Autodesk Inventor part; units mm, degrees
ref_plane "YZ Plane" through (0, 0, 0) normal (1, 0, 0) x (0, 1, 0)
ref_plane "XZ Plane" through (0, 0, 0) normal (0, 1, 0) x (-1, 0, 0)
ref_plane "XY Plane" through (0, 0, 0) normal (0, 0, 1) x (1, 0, 0)
sketch "Sketch2" plane through (0, 0, 0) normal (1, 0, 0) x (0, 1, 0)
  line L0 (0, -0.635) -> (0, -31.75)
  line L1 (0, -31.75) -> (41.275, -31.75)
  line L2 (41.275, -31.75) -> (41.275, -6.35)
  line L3 (41.275, -6.35) -> (104.775, -6.35)
  line L4 (104.775, -6.35) -> (104.775, -1.0105)
  line L5 (104.775, 0) -> (0, 0)
  line L6 (-2.54, 0) -> (-2.54, -0.635)
  line L7 (-2.54, -0.635) -> (0, -0.635)
  line L8 (-2.54, 0) -> (0, 0)
  line L9 (104.775, 0) -> (150.2763, 0)
  line L10 (150.2763, 0) -> (150.2763, -1.0105)
  line L11 (150.2763, -1.0105) -> (104.775, -1.0105)
  dimension "d0" = 41.275
  dimension "d1" = 63.5
  dimension "d2" = 31.75
  dimension "d3" = 6.35
  dimension "d8" = 2.54
  dimension "d9" = 0.635
revolve "Revolution1" add sketch "Sketch2" angle 360 about axis through (0, 104.775, 0) along (0, -1, 0)
chamfer "Chamfer1" distance 1.27 angle 45 2 edges at (0, 41.275, 31.75) (0, 0, 31.75)
properties part number "Fixture_Weight"
The model under review builds one solid part; all positions refer to its coordinate system, in mm. A direction names the side the tool comes from. Round coordinates to 2 decimals unless told otherwise and drop trailing zeros. Loops run counter-clockwise (first coordinate to the right, second up) from the corner with the lowest first, then second, coordinate; pieces in that order, holes last. Notation, with made-up numbers: M -7.5,20.25 L 34.5,20.25 A11 cw 34.5,32.25 Z; hole C -1.5,54 d9. An arc over 180 degrees is marked long. Answer as a JSON object with one key per item and string values.
Item 1: Tool access review of faces 1 (the face through (6.2, 73.47, 1.38)), 2 (the face through (30.995, 20.909, 6.883)): name each direction out of +Z, -Z, +X, -X, +Y, -Y from which nothing blocks a thin tool from reaching the whole face with its end or side.
Check sheet entries:
{"face 1": "+Y", "face 2": "+Y, -Y"}
Item 2: We need section B-B, the plane y = 135.5. State the section outline as (x, z) points, and give its area (3 significant figures).
Check sheet entries:
{"outline": "C 0,0 d2.02", "area": "3.21 mm2"}
Item 3: For line 1 along Y through (x, z) = (-7, -3) (3 decimals); line 2 along X through (y, z) = (22, 1); line 3 along Z through (x, y) = (-4, 28), list the stretches that pass through material, from the lowest coordinate up.
Check sheet entries:
{"line 1": "0 to 41.275", "line 2": "-31.73 to 31.73", "line 3": "-31.5 to 31.5"}
Item 4: We need section A-A, the plane y = 24. State the section outline as (x, z) points, and give its area (3 significant figures).
Check sheet entries:
{"outline": "C 0,0 d63.5", "area": "3,170 mm2"}
Item 5: Clearance check with flat-ended pins moving along their axes: P1, Ø4, axis at x = -7, z = 24, coming from the +Y side (3 decimals); P2, Ø8, axis at y = 15.5, z = -23.5, coming from the +X side; P3, Ø10, axis at x = 3, z = 1, coming from the +Y side; P4, Ø3, axis at y = 29, z = 14, coming from the +X side. State where each tip first meets the part, or that it passes through.
Check sheet entries:
{"P1": "y = 41.275", "P2": "x = 25.06", "P3": "y = 150.28", "P4": "x = 29.19"}
